Autodesk Inventor part; units mm, degrees
ref_plane "YZ Plane" through (0, 0, 0) normal (1, 0, 0) x (0, 1, 0)
ref_plane "XZ Plane" through (0, 0, 0) normal (0, 1, 0) x (-1, 0, 0)
ref_plane "XY Plane" through (0, 0, 0) normal (0, 0, 1) x (1, 0, 0)
sketch "2020_Base" plane through (0, 0, 0) normal (0, 1, 0) x (-1, 0, 0)
  line L0 (2307.7639, 1192.1343) -> (2307.7639, 1195.3915)
  arc A0 (2307.7639, 1195.3915) -> (2307.4639, 1195.6915) centre (2307.4639, 1195.3915) ccw
  line L1 (2307.4639, 1195.6915) -> (2306.5639, 1195.6915)
  arc A1 (2306.2639, 1195.9915) -> (2306.5639, 1195.6915) centre (2306.5639, 1195.9915) ccw
  line L2 (2306.2639, 1195.9915) -> (2306.2639, 1196.8915)
  arc A2 (2306.5639, 1197.1915) -> (2306.2639, 1196.8915) centre (2306.5639, 1196.8915) ccw
  line L3 (2306.5639, 1197.1915) -> (2313.3139, 1197.1915)
  arc A3 (2313.6139, 1196.8915) -> (2313.3139, 1197.1915) centre (2313.3139, 1196.8915) ccw
  line L4 (2313.6139, 1196.8915) -> (2313.6139, 1190.1415)
  arc A4 (2313.3139, 1189.8415) -> (2313.6139, 1190.1415) centre (2313.3139, 1190.1415) ccw
  line L5 (2313.3139, 1189.8415) -> (2312.4139, 1189.8415)
  arc A5 (2312.1139, 1190.1415) -> (2312.4139, 1189.8415) centre (2312.4139, 1190.1415) ccw
  line L6 (2312.1139, 1190.1415) -> (2312.1139, 1191.0415)
  arc A6 (2312.1139, 1191.0415) -> (2311.8139, 1191.3415) centre (2311.8139, 1191.0415) ccw
  line L7 (2311.8139, 1191.3415) -> (2308.5567, 1191.3415)
  arc A7 (2308.5567, 1191.3415) -> (2308.3217, 1191.2281) centre (2308.5567, 1191.0415) ccw
  arc A8 (2308.3217, 1191.2281) -> (2306.9212, 1187.4988) centre (2313.4048, 1187.1915) ccw
  line L8 (2306.9212, 1187.4988) -> (2306.6139, 1187.1915)
  line L9 (2306.6139, 1187.1915) -> (2306.9212, 1186.8843)
  arc A9 (2306.9212, 1186.8843) -> (2308.3217, 1183.155) centre (2313.4048, 1187.1915) ccw
  arc A10 (2308.3217, 1183.155) -> (2308.5567, 1183.0415) centre (2308.5567, 1183.3415) ccw
  line L10 (2308.5567, 1183.0415) -> (2311.8139, 1183.0415)
  arc A11 (2311.8139, 1183.0415) -> (2312.1139, 1183.3415) centre (2311.8139, 1183.3415) ccw
  line L11 (2312.1139, 1183.3415) -> (2312.1139, 1184.2415)
  arc A12 (2312.4139, 1184.5415) -> (2312.1139, 1184.2415) centre (2312.4139, 1184.2415) ccw
  line L12 (2312.4139, 1184.5415) -> (2313.3139, 1184.5415)
  arc A13 (2313.6139, 1184.2415) -> (2313.3139, 1184.5415) centre (2313.3139, 1184.2415) ccw
  line L13 (2313.6139, 1184.2415) -> (2313.6139, 1177.4915)
  arc A14 (2313.3139, 1177.1915) -> (2313.6139, 1177.4915) centre (2313.3139, 1177.4915) ccw
  line L14 (2313.3139, 1177.1915) -> (2306.5639, 1177.1915)
  arc A15 (2306.2639, 1177.4915) -> (2306.5639, 1177.1915) centre (2306.5639, 1177.4915) ccw
  line L15 (2306.2639, 1177.4915) -> (2306.2639, 1178.3915)
  arc A16 (2306.5639, 1178.6915) -> (2306.2639, 1178.3915) centre (2306.5639, 1178.3915) ccw
  line L16 (2306.5639, 1178.6915) -> (2307.4639, 1178.6915)
  arc A17 (2307.4639, 1178.6915) -> (2307.7639, 1178.9915) centre (2307.4639, 1178.9915) ccw
  line L17 (2307.7639, 1178.9915) -> (2307.7639, 1182.2488)
  arc A18 (2307.7639, 1182.2488) -> (2307.6505, 1182.4837) centre (2307.4639, 1182.2488) ccw
  arc A19 (2307.6505, 1182.4837) -> (2303.9212, 1183.8843) centre (2303.6139, 1177.4007) ccw
  line L18 (2303.9212, 1183.8843) -> (2303.6139, 1184.1915)
  line L19 (2303.6139, 1184.1915) -> (2303.3066, 1183.8843)
  arc A20 (2303.3066, 1183.8843) -> (2299.5774, 1182.4837) centre (2303.6139, 1177.4007) ccw
  arc A21 (2299.5774, 1182.4837) -> (2299.4639, 1182.2488) centre (2299.7639, 1182.2488) ccw
  line L20 (2299.4639, 1182.2488) -> (2299.4639, 1178.9915)
  arc A22 (2299.4639, 1178.9915) -> (2299.7639, 1178.6915) centre (2299.7639, 1178.9915) ccw
  line L21 (2299.7639, 1178.6915) -> (2300.6639, 1178.6915)
  arc A23 (2300.9639, 1178.3915) -> (2300.6639, 1178.6915) centre (2300.6639, 1178.3915) ccw
  line L22 (2300.9639, 1178.3915) -> (2300.9639, 1177.4915)
  arc A24 (2300.6639, 1177.1915) -> (2300.9639, 1177.4915) centre (2300.6639, 1177.4915) ccw
  line L23 (2300.6639, 1177.1915) -> (2293.9139, 1177.1915)
  arc A25 (2293.6139, 1177.4915) -> (2293.9139, 1177.1915) centre (2293.9139, 1177.4915) ccw
  line L24 (2293.6139, 1177.4915) -> (2293.6139, 1184.2415)
  arc A26 (2293.9139, 1184.5415) -> (2293.6139, 1184.2415) centre (2293.9139, 1184.2415) ccw
  line L25 (2293.9139, 1184.5415) -> (2294.8139, 1184.5415)
  arc A27 (2295.1139, 1184.2415) -> (2294.8139, 1184.5415) centre (2294.8139, 1184.2415) ccw
  line L26 (2295.1139, 1184.2415) -> (2295.1139, 1183.3415)
  arc A28 (2295.1139, 1183.3415) -> (2295.4139, 1183.0415) centre (2295.4139, 1183.3415) ccw
  line L27 (2295.4139, 1183.0415) -> (2298.6712, 1183.0415)
  arc A29 (2298.6712, 1183.0415) -> (2298.9061, 1183.155) centre (2298.6712, 1183.3415) ccw
  arc A30 (2298.9061, 1183.155) -> (2300.3066, 1186.8843) centre (2293.8231, 1187.1915) ccw
  line L28 (2300.3066, 1186.8843) -> (2300.6139, 1187.1915)
  line L29 (2300.6139, 1187.1915) -> (2300.3066, 1187.4988)
  arc A31 (2300.3066, 1187.4988) -> (2298.9061, 1191.2281) centre (2293.8231, 1187.1915) ccw
  arc A32 (2298.9061, 1191.2281) -> (2298.6712, 1191.3415) centre (2298.6712, 1191.0415) ccw
  line L30 (2298.6712, 1191.3415) -> (2295.4139, 1191.3415)
  arc A33 (2295.4139, 1191.3415) -> (2295.1139, 1191.0415) centre (2295.4139, 1191.0415) ccw
  line L31 (2295.1139, 1191.0415) -> (2295.1139, 1190.1415)
  arc A34 (2294.8139, 1189.8415) -> (2295.1139, 1190.1415) centre (2294.8139, 1190.1415) ccw
  line L32 (2294.8139, 1189.8415) -> (2293.9139, 1189.8415)
  arc A35 (2293.6139, 1190.1415) -> (2293.9139, 1189.8415) centre (2293.9139, 1190.1415) ccw
  line L33 (2293.6139, 1190.1415) -> (2293.6139, 1196.8915)
  arc A36 (2293.9139, 1197.1915) -> (2293.6139, 1196.8915) centre (2293.9139, 1196.8915) ccw
  line L34 (2293.9139, 1197.1915) -> (2300.6639, 1197.1915)
  arc A37 (2300.9639, 1196.8915) -> (2300.6639, 1197.1915) centre (2300.6639, 1196.8915) ccw
  line L35 (2300.9639, 1196.8915) -> (2300.9639, 1195.9915)
  arc A38 (2300.6639, 1195.6915) -> (2300.9639, 1195.9915) centre (2300.6639, 1195.9915) ccw
  line L36 (2300.6639, 1195.6915) -> (2299.7639, 1195.6915)
  arc A39 (2299.7639, 1195.6915) -> (2299.4639, 1195.3915) centre (2299.7639, 1195.3915) ccw
  line L37 (2299.4639, 1195.3915) -> (2299.4639, 1192.1343)
  arc A40 (2299.4639, 1192.1343) -> (2299.5774, 1191.8994) centre (2299.7639, 1192.1343) ccw
  arc A41 (2299.5774, 1191.8994) -> (2303.3066, 1190.4988) centre (2303.6139, 1196.9824) ccw
  line L38 (2303.3066, 1190.4988) -> (2303.6139, 1190.1915)
  line L39 (2303.6139, 1190.1915) -> (2303.9212, 1190.4988)
  arc A42 (2303.9212, 1190.4988) -> (2307.6505, 1191.8994) centre (2303.6139, 1196.9824) ccw
  arc A43 (2307.6505, 1191.8994) -> (2307.7639, 1192.1343) centre (2307.4639, 1192.1343) ccw
  circle A44 centre (2310.6139, 1194.1915) radius 2
  circle A45 centre (2303.6139, 1187.1915) radius 2.15
  circle A46 centre (2296.6139, 1194.1915) radius 2
  circle A47 centre (2296.6139, 1180.1915) radius 2
  circle A48 centre (2310.6139, 1180.1915) radius 2
  point P0 (0, 0)
extrude "300mm 2020" add sketch "2020_Base" along normal blind 250
properties part number "100mm 2020" material "알루미늄 6061"
Design review of the part built by this model. Coordinates are the model's own, in mm. Give positions to 0.01 mm unless a question says otherwise; leave off trailing zeros. One line per item, written item: value.
Q1. We need section A-A on y = 134. Give the number of separate pieces and of enclosed holes in the cut face, and give its area (3 significant figures).
Numbers:
separate pieces: 1
enclosed holes: 5
area: 146 mm^2
Q2. For L1, parallel to Z at x = -2296.75, y = 197; L2, parallel to X at y = 67, z = 1180; L3, parallel to Z at x = -2303.25, y = 210, list the stretches that pass through material, from the lowest coordinate up.
Numbers:
L1: z = 1177.19 to 1178.2, 1182.19 to 1183.04, 1191.34 to 1192.2, 1196.19 to 1197.19
L2: x = -2313.61 to -2312.6, -2308.62 to -2307.76, -2299.46 to -2298.6, -2294.62 to -2293.61
L3: z = 1183.88 to 1185.07, 1189.31 to 1190.5
Q3. Draft analysis for pull direction X (two halves, no side actions). For faces 1 (the flat face through (-2301, 250, 1187)), 2 (the flat face through (-2293.614, 123, 1181)), 3 (the cylindrical face through (-2311.537, 123.25, 1181.966)), state which applies: pulls with the +X half, pulls with the -X half, needs draft (parallel to the pull), parting line crosses it, or undercut.
Numbers:
face 1: needs draft
face 2: pulls with the +X half
face 3: undercut
